```python
from build123d import *

# Parameters (mm, degrees)
EXTRUDE1_DEPTH      = 4
EXTRUDE2_DEPTH      = 12.357816692
EXTRUDE2_DEPTH_BACK = 12.357816692
SKETCH2_R           = 1
EXTRUDE3_DEPTH      = 12.357816692
EXTRUDE3_DEPTH_BACK = 12.357816692
SKETCH4_W           = 6
SKETCH4_H           = 8.732029078
FILLET2_R           = 1
EXTRUDE4_DEPTH      = 14
EXTRUDE4_DEPTH_BACK = 3
SKETCH3_R           = 1.5
EXTRUDE5_DEPTH      = 9
SKETCH6_R           = 1.5
EXTRUDE6_DEPTH      = 1
SKETCH7_R           = 0.6
EXTRUDE7_DEPTH      = 1
FILLET3_R           = 1
SKETCH8_R           = 2
EXTRUDE8_DEPTH      = 1
SKETCH9_R           = 15.158662045
EXTRUDE9_DEPTH      = 18.811513131


with BuildPart() as part:
    # Sketch1 → Extrude1 (new, symmetric)
    with BuildSketch(Plane.XY):
        Polygon((0, 0), (-7, 0), (-7, 8), (7, 8), (7, 0), align=None)
    extrude(amount=EXTRUDE1_DEPTH, both=True)

    # Sketch2 → Extrude2 (cut, two sides: drawn at the far end of the back side and taken through both)
    with BuildSketch(Plane.XY.offset(-EXTRUDE2_DEPTH_BACK)):
        with Locations((4.5, 5.5)):
            Circle(SKETCH2_R)
    extrude(amount=EXTRUDE2_DEPTH + EXTRUDE2_DEPTH_BACK, mode=Mode.SUBTRACT)

    # Sketch4 → Extrude3 (cut, two sides: drawn at the far end of the back side and taken through both)
    with BuildSketch(Plane(origin=(0, 0, 0), x_dir=(0, 0, -1), z_dir=(1, 0, 0)).offset(-EXTRUDE3_DEPTH_BACK)):
        with Locations((0, 5.366014539)):
            Rectangle(SKETCH4_W, SKETCH4_H)
    extrude(amount=EXTRUDE3_DEPTH + EXTRUDE3_DEPTH_BACK, mode=Mode.SUBTRACT)

    # Fillet2
    fillet2_edges = [part.edges().sort_by_distance(p)[0] for p in [
        (-7, 8, -3.5),
        (7, 8, -3.5),
        (-7, 8, 3.5),
        (7, 8, 3.5),
    ]]
    fillet(fillet2_edges, radius=FILLET2_R)

    # Sketch3 → Extrude4 (add, two sides: drawn at the far end of the back side and taken through both)
    with BuildSketch(Plane.XY.offset(-EXTRUDE4_DEPTH_BACK)):
        with Locations((-3, 4.5)):
            Circle(SKETCH3_R)
    extrude(amount=EXTRUDE4_DEPTH + EXTRUDE4_DEPTH_BACK)

    # Sketch5 → Extrude5 (cut)
    with BuildSketch(Plane.XY.offset(14)):
        Polygon((-4, 4.5), (-4, 6.060686456), (-4.95644391, 6.060686456), (-4.95644391, 2.5), (-4, 2.5), align=None)
    extrude(amount=-EXTRUDE5_DEPTH, mode=Mode.SUBTRACT)

    # Sketch6 → Extrude6 (add)
    with BuildSketch(Plane.XZ):
        with Locations((-7, 0)):
            Circle(SKETCH6_R)
        with Locations((7, 0)):
            Circle(SKETCH6_R)
    extrude(amount=-EXTRUDE6_DEPTH)

    # Sketch7 → Extrude7 (cut)
    with BuildSketch(Plane.XZ):
        with Locations((-7, 0)):
            Circle(SKETCH7_R)
        with Locations((7, 0)):
            Circle(SKETCH7_R)
    extrude(amount=-EXTRUDE7_DEPTH, mode=Mode.SUBTRACT)

    # Fillet3
    fillet3_edges = [part.edges().sort_by_distance(p)[0] for p in [
        (7, 0.5, -1.5),
        (7, 0.5, 1.5),
        (-7, 0.5, 1.5),
        (-7, 0.5, -1.5),
    ]]
    fillet(fillet3_edges, radius=FILLET3_R)

    # Sketch8 → Extrude8 (cut)
    with BuildSketch(Plane.XZ):
        Circle(SKETCH8_R)
    extrude(amount=-EXTRUDE8_DEPTH, mode=Mode.SUBTRACT)

    # Sketch9 → Extrude9 (cut, through all)
    with BuildSketch(Plane(origin=(0, 1, 0), x_dir=(1, 0, 0), z_dir=(0, 1, 0))):
        Circle(SKETCH9_R)
    extrude(amount=EXTRUDE9_DEPTH, mode=Mode.SUBTRACT)


solid = part.part
```
For this review, take the finished solid that the model builds, in its own axes (mm). A direction names the side the tool comes from. Round coordinates to 2 decimals unless told otherwise and drop trailing zeros. Write each loop counter-clockwise with the first axis right and the second up, starting at its lowest first coordinate (ties: lowest second). Pieces come first, ordered by that corner, then holes. Notation, with made-up numbers: (51, 52.5) - (100, 52.5) arc R15 ccw to (100, 66.5) - close; hole circle Ø7 at (23, -7.5). An arc over 180 degrees is marked (long way). Write each question's results on one line, items separated by ' | '.
Item 1: Take a section at B-B on y = 0.6. State the section outline as (x, z) points, then the cut area to 3 significant figures.
Calculated:
outline: (-7.6, -1.37) arc R1 cw to (-7, -2.29) - (-7, -4) - (7, -4) - (7, -2.29) arc R1 cw to (7.6, -1.37) arc R1.5 ccw to (7.6, 1.37) arc R1 cw to (7, 2.29) - (7, 4) - (-7, 4) - (-7, 2.29) arc R1 cw to (-7.6, 1.37) arc R1.5 ccw to start; hole circle Ø1.2 at (-7, 0); hole circle Ø4 at (0, 0); hole circle Ø1.2 at (7, 0) | area: 105 mm^2
Item 2: Draft analysis for pull direction Z (two halves, no side actions). For faces 1 (the face through (-8.5, 0.5, 0)), 2 (the face through (-2, 1, 1)), 3 (the face through (-0.434, 0.493, -1.952)), state which applies: pulls with the +Z half, pulls with the -Z half, needs draft (parallel to the pull), parting line crosses it, or undercut.
Calculated:
face 1: parting line crosses it | face 2: needs draft | face 3: undercut
Item 3: To check wall thickness, follow line 1 along X through (y, z) = (0.65, -0.25); line 2 along X through (y, z) = (0.2, 1.75); line 3 along Z through (x, y) = (1.75, 0.2). State the ranges of each line that lie inside material, in increasing order. Write a range as from..to.
Calculated:
line 1: x = -8.48..-7.55, -6.45..-1.98, 1.98..6.45, 7.55..8.48 | line 2: x = -7.16..-0.97, 0.97..7.16 | line 3: z = -4..-0.97, 0.97..4
Item 4: Take a section at C-C on x = 0. State the section outline as (y, z) points, then the cut area to 3 significant figures.
Calculated:
outline: (0, -4) - (1, -4) - (1, -2) - (0, -2) - close; (0, 2) - (1, 2) - (1, 4) - (0, 4) - close | area: 4.00 mm^2
Item 5: Take a section at A-A on z = 0. State the section outline as (x, y) points.
Calculated:
outline: (-8.5, 0) - (-7.6, 0) - (-7.6, 1) - (-8.5, 1) - close; (-6.4, 0) - (-2, 0) - (-2, 1) - (-6.4, 1) - close; (2, 0) - (6.4, 0) - (6.4, 1) - (2, 1) - close; (7.6, 0) - (8.5, 0) - (8.5, 1) - (7.6, 1) - close
Item 6: For pin 1 (0.5 mm diameter, centred on y = 0.5, z = 3, fed in from -X), flat-tipped, find the tip position at first contact; note if it passes through.
Calculated:
pin 1: stops at x = -7
Item 7: For faces 4 (the face through (7, 0.5, -3.1)), 5 (the face through (-7, 0.5, 3.2)), 6 (the face through (-7, 0.5, -3.1)), 7 (the face through (7, 0.5, 3.2)), list the 3-axis set-ups (+Z, -Z, +X, -X, +Y, -Y) from which the entire face can be reached by the end or side of a thin tool; tool diameter is ignored.
Calculated:
face 4: -Z, +X, +Y, -Y | face 5: +Z, -X, +Y, -Y | face 6: -Z, -X, +Y, -Y | face 7: +Z, +X, +Y, -Y
